```python
from build123d import *

# Parameters (mm, degrees)
F1_DEPTH      = 25
F1_DEPTH_BACK = 25
F2_W          = 8
F2_H          = 10
F3_DEPTH      = 30
F0_W          = 13
F0_H          = 10
F0_W_2        = 18
F0_H_2        = 20
F4_DEPTH      = 10
F4_DEPTH_BACK = 10


with BuildPart() as f1:
    # F0 (on Front) → F1 (new body, two sides)
    with BuildSketch(Plane.XZ) as f1_sk:
        with BuildLine():
            ThreePointArc((20, 55), (0, 75), (-20, 55))
            Line((-20, 55), (20, 55))
        make_face()
        with BuildLine():
            Line((20, 55), (-20, 55))
            ThreePointArc((-20, 55), (0, 35), (20, 55))
        make_face()
        with BuildLine():
            Line((-40, 55), (-40, 0))
            Line((-40, 0), (40, 0))
            Line((40, 0), (40, 20))
            Line((40, 20), (40, 55))
            Line((40, 55), (27, 55))
            Line((27, 55), (20, 55))
            ThreePointArc((20, 55), (0, 35), (-20, 55))
            Line((-20, 55), (-27, 55))
            Line((-27, 55), (-40, 55))
        make_face()
    extrude(amount=F1_DEPTH)
    extrude(f1_sk.sketch, amount=-F1_DEPTH_BACK)

    # F2 (on face) → F3 (cut)
    with BuildSketch(Plane.XZ.offset(25)):
        with BuildLine():
            Line((22.0221508968, 90.4806110974), (-22.9720887471, 90.4806110974))
            Line((-22.9720887471, 90.4806110974), (-22.9720887471, 65))
            Line((-22.9720887471, 65), (-17.3205080757, 65))
            ThreePointArc((-17.3205080757, 65), (0, 75), (17.3205080757, 65))
            Line((17.3205080757, 65), (22.0221508968, 65))
            Line((22.0221508968, 65), (22.0221508968, 90.4806110974))
        make_face()
        with BuildLine():
            ThreePointArc((17.3205080757, 65), (0, 75), (-17.3205080757, 65))
            Line((-17.3205080757, 65), (-8, 65))
            Line((-8, 65), (0, 65))
            Line((0, 65), (8, 65))
            Line((8, 65), (17.3205080757, 65))
        make_face()
        with Locations((4, 60)):
            Rectangle(F2_W, F2_H)
        with Locations((-4, 60)):
            Rectangle(F2_W, F2_H)
    extrude(amount=-F3_DEPTH, mode=Mode.SUBTRACT)

    # F0 (on Front) → F4 (join, two sides)
    with BuildSketch(Plane.XZ) as f4_sk:
        Polygon((-58, 0), (-40, 0), (-40, 55), (-27, 55), (-27, 65), (-40, 65), (-58, 20), align=None)
        Polygon((40, 55), (40, 20), (58, 20), (40, 65), align=None)
        with Locations((33.5, 60)):
            Rectangle(F0_W, F0_H)
        with Locations((49, 10)):
            Rectangle(F0_W_2, F0_H_2)
    extrude(amount=F4_DEPTH)
    extrude(f4_sk.sketch, amount=-F4_DEPTH_BACK)


solid = f1.part
```
Here's how the part is built. I have some questions about the finished solid (model axes, mm). A direction names the side the tool comes from. Give positions to 0.01 mm unless a question says otherwise; leave off trailing zeros. Order: outer loops, then holes, each group sorted by start corner. A loop starts at its lowest first (then second) coordinate and runs counter-clockwise, first axis right, second up. Notation, with made-up numbers: M 64,-19 L 104,-19 A18 ccw 104,-15 Z; hole C 70.25,29.25 d8. An arc over 180 degrees is marked long. Use a Markdown table: item, result. Add a question column.
1. Suppose I cut it at B-B (z = 22.5). List the corners of the cut face in (x, y) for me, and give its area (3 significant figures).
2. Suppose I cut it at C-C (x = 30.5). List the corners of the cut face in (y, z) for me, and give its area (3 significant figures).
3. If we mould it in two halves opening along X, with no side actions, what happens to faces 1 (the flat face through (-46, 10, 26)), 2 (the flat face through (-48.87, -0.14, 42.82)), 3 (the flat face through (-8, -10, 60))? For each: +X half, -X half, draft (parallel to the pull), parting line (faces both ways), or undercut.
4. Suppose I cut it at D-D (y = 2). List the corners of the cut face in (x, z) for me.
5. For pin 1 Ø2 at (y, z) = (19, 11) entering from -X; pin 2 Ø6 at (y, z) = (12.5, 62) entering from -X; pin 3 Ø22 at (x, y) = (30.5, 8.5) entering from +Z, each with a flat end and sliding along its axis, tell me the tip position at first contact or that it passes through.
6. I need wall thicknesses on probe 1 along X at (y, z) = (-8, 64.5); probe 2 along X at (y, z) = (-7.5, 55.5); probe 3 along Y at (x, z) = (-50.5, 5.5). Which ranges of each line are inside material? Lowest first, please. Write a range as from..to.
7. Suppose I cut it at A-A (y = -16.5). List the corners of the cut face in (x, z) for me.
8. On a 3-axis mill with a long thin cutter (end or side, diameter ignored), from which of +Z, -Z, +X, -X, +Y, -Y can I reach the whole of each face in a straight line? I mean faces 4 (the flat face through (27, 0, 60)), 5 (the flat face through (0, -10, 55)), 6 (the flat face through (-33, 0, 65)). Say none if no direction works.
Results list:
| question | item | result |
|---|---|---|
| 1 | outline | M -57,-10 L -40,-10 L -40,-25 L 40,-25 L 40,-10 L 57,-10 L 57,10 L 40,10 L 40,25 L -40,25 L -40,10 L -57,10 Z |
| 1 | area | 4,680 mm² |
| 2 | outline | M -25,0 L 25,0 L 25,55 L 10,55 L 10,65 L -10,65 L -10,55 L -25,55 Z |
| 2 | area | 2,950 mm² |
| 3 | face 1 | draft |
| 3 | face 2 | -X half |
| 3 | face 3 | undercut |
| 4 | outline | M -58,0 L 58,0 L 58,20 L 40,65 L 27,65 L 27,55 L 20,55 A20 ccw 17.32,65 L 8,65 L 8,55 L -8,55 L -8,65 L -17.32,65 A20 ccw -20,55 L -27,55 L -27,65 L -40,65 L -58,20 Z |
| 5 | pin 1 | stops at x = -40 |
| 5 | pin 2 | stops at x = -41.86 |
| 5 | pin 3 | stops at z = 65 |
| 6 | probe 1 | x = -40.2..-27, -17.6..-8, 8..17.6, 27..40.2 |
| 6 | probe 2 | x = -43.8..-27, -19.99..-8, 8..19.99, 27..43.8 |
| 6 | probe 3 | y = -10..10 |
| 7 | outline | M -40,0 L 40,0 L 40,55 L 20,55 A20 ccw 17.32,65 L 8,65 L 8,55 L -8,55 L -8,65 L -17.32,65 A20 ccw -20,55 L -40,55 Z |
| 8 | face 4 | +Z, +Y, -Y |
| 8 | face 5 | +Z, -Y |
| 8 | face 6 | +Z, -X, +Y, -Y |
